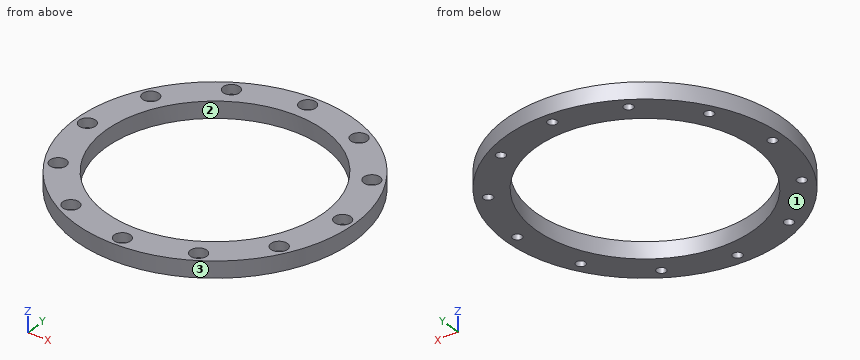
from build123d import *

# Parameters (mm, degrees)
SKETCH_1_R                = 51
EXTRUDE_1_DEPTH           = 6
HOLE_WIZARD_1_D           = 3.4
HOLE_WIZARD_1_CBORE_D     = 6
HOLE_WIZARD_1_CBORE_DEPTH = 3.4
SKETCH_4_R                = 40
CUT_EXTRUDE_1_DEPTH       = 73.374028491
PATTERN_CIRCULAR_1_COUNT  = 12


with BuildPart() as part:
    # 草图1 → 凸台-拉伸1 (new body)
    with BuildSketch(Plane.XY):
        Circle(SKETCH_1_R)
    extrude(amount=EXTRUDE_1_DEPTH)

    # 打孔尺寸(%根据)内六角圆柱头螺钉的类型1 (through all)
    with Locations(Plane.XY.offset(6)):
        with Locations((0, 46.75)):
            hole_wizard_1 = CounterBoreHole(HOLE_WIZARD_1_D / 2, HOLE_WIZARD_1_CBORE_D / 2, HOLE_WIZARD_1_CBORE_DEPTH)

    # 草图4 → 切除-拉伸1 (cut, through all)
    with BuildSketch(Plane.XY.offset(6)):
        Circle(SKETCH_4_R)
    extrude(amount=-CUT_EXTRUDE_1_DEPTH, mode=Mode.SUBTRACT)

    # 阵列(圆周)1: 打孔尺寸(%根据)内六角圆柱头螺钉的类型1 ×12 about axis
    pattern_circular_1_axis = Axis((0, 0, 0), (0, 0, 1))
    for i in range(1, PATTERN_CIRCULAR_1_COUNT):
        add(hole_wizard_1.rotate(pattern_circular_1_axis, i * 360 / PATTERN_CIRCULAR_1_COUNT), mode=Mode.SUBTRACT)


solid = part.part
The listing builds one solid part. Answer for the finished solid, in the listing's coordinates (mm). Face numbers are marked on the shaded views. Give positions to 0.01 mm unless a question says otherwise; leave off trailing zeros. Loops run counter-clockwise (first coordinate to the right, second up) from the corner with the lowest first, then second, coordinate; pieces in that order, holes last. Notation, with made-up numbers: (46.5, 62) - (57.5, 62) arc R23 cw to (57.5, 83) - close; hole circle Ø7 at (51.25, -12). An arc over 180 degrees is marked (long way). Answer as a JSON object with one key per item and string values.
1. Flat-ended cylindrical pins translate along their axes: pin 1 Ø5.5 at (x, y) = (0, 46.75) entering from +Z; pin 2 Ø1 at (x, z) = (40.5, 5.5) entering from -Y; pin 3 Ø1.5 at (y, z) = (-28, 4.5) entering from +X. Find the tip coordinate at first contact, or state that the pin passes through.
Determined:
{"pin 1": "z = 2.6", "pin 2": "y = -31.64", "pin 3": "x = 43.11"}
2. A cutting plane is placed at D-D (x = 11). Write down the section's boundary in (y, z), then the cut area to 3 significant figures.
Determined:
{"outline": "(-49.8, 0) - (-38.46, 0) - (-38.46, 6) - (-49.8, 6) - close; (38.46, 0) - (49.8, 0) - (49.8, 6) - (38.46, 6) - close", "area": "136 mm²"}
3. A cutting plane is placed at B-B (y = 46.75). Write down the section's boundary in (x, z), then the cut area to 3 significant figures.
Determined:
{"outline": "(-20.38, 0) - (-1.7, 0) - (-1.7, 2.6) - (-3, 2.6) - (-3, 6) - (-20.38, 6) - close; (1.7, 0) - (20.38, 0) - (20.38, 6) - (3, 6) - (3, 2.6) - (1.7, 2.6) - close", "area": "215 mm²"}
4. Find the intervals of material crossed by L1, parallel to Y at x = 0, z = 1.9; L2, parallel to Y at x = -0.5, z = 2.75; L3, parallel to Y at x = -8, z = 2.7, in increasing order. Write a range as [from, to].
Determined:
{"L1": "[-51, -48.45], [-45.05, -40], [40, 45.05], [48.45, 51]", "L2": "[-51, -49.71], [-43.79, -40], [40, 43.79], [49.71, 51]", "L3": "[-50.37, -39.19], [39.19, 50.37]"}
5. A cutting plane is placed at C-C (z = 3.95). Give the number of separate pieces and of enclosed holes in the cut face, then the cut area to 3 significant figures.
Determined:
{"separate pieces": "1", "enclosed holes": "13", "area": "2,810 mm²"}
6. A cutting plane is placed at A-A (x = 0). Write down the section's boundary in (y, z).
Determined:
{"outline": "(-51, 0) - (-48.45, 0) - (-48.45, 2.6) - (-49.75, 2.6) - (-49.75, 6) - (-51, 6) - close; (-45.05, 0) - (-40, 0) - (-40, 6) - (-43.75, 6) - (-43.75, 2.6) - (-45.05, 2.6) - close; (40, 0) - (45.05, 0) - (45.05, 2.6) - (43.75, 2.6) - (43.75, 6) - (40, 6) - close; (48.45, 0) - (51, 0) - (51, 6) - (49.75, 6) - (49.75, 2.6) - (48.45, 2.6) - close"}
7. For a pull along Y with two mould halves and no side action, classify the marked faces 1, 2 and 3 as pulls with the +Y half, pulls with the -Y half, needs draft (parallel to the pull), parting line crosses it, or undercut.
Determined:
{"face 1": "needs draft", "face 2": "undercut", "face 3": "parting line crosses it"}
